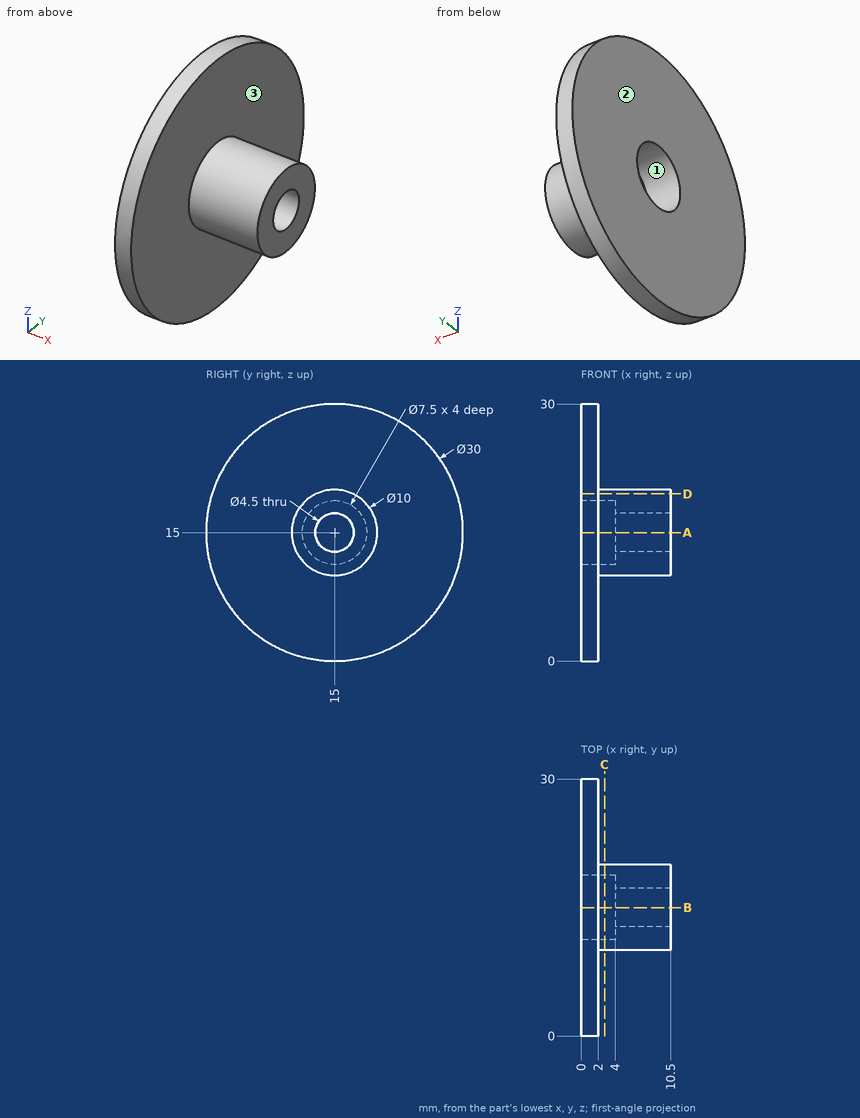
Input: dimensioned drawing with shaded views. Units: mm. Origin: part minimum x, y, z. A direction names the side the tool comes from. Give positions to 0.01 mm unless a question says otherwise; leave off trailing zeros. Order: outer loops, then holes, each group sorted by start corner. A loop starts at its lowest first (then second) coordinate and runs counter-clockwise, first axis right, second up. Notation, with made-up numbers: (-19, 14.5) -> (23, 14.5) arc R22 ccw to (23, 22.5) -> close; hole circle Ø2 at (-24, 2). An arc over 180 degrees is marked (long way). Answer as a JSON object with one key per item and string values.
Q1. First-contact query: pin 1 (1.5 mm diameter, centred on x = 2, y = 5, fed in from +Z); pin 2 (6 mm diameter, centred on x = 4, z = 7, fed in from +Y); pin 3 (5 mm diameter, centred on y = 15, z = 15, fed in from -X); pin 4 (1.5 mm diameter, centred on x = 6, y = 21.5, fed in from +Z). Flat tips, straight axial feed; report the tip coordinate or a pass-through.
Entries:
{"pin 1": "stops at z = 26.81", "pin 2": "stops at y = 28.85", "pin 3": "stops at x = 4", "pin 4": "passes through"}
Q2. Section D-D (z = 19.5). Output: boundary loops of the cut face in (x, y), plus the area to 3 significant figures.
Entries:
{"outline": "(0, 0.69) -> (2, 0.69) -> (2, 12.82) -> (10.5, 12.82) -> (10.5, 17.18) -> (2, 17.18) -> (2, 29.31) -> (0, 29.31) -> close", "area": "94.3 mm^2"}
Q3. Access query for the marked faces 1, 2 and 3. Directions: +Z, -Z, +X, -X, +Y, -Y. A direction counts if a zero-diameter tool reaches every point of the face in a straight line with its end or side. Return the directions, or none.
Entries:
{"face 1": "-X", "face 2": "+Z, -Z, -X, +Y, -Y", "face 3": "+X"}
Q4. Section A-A (z = 15). Output: boundary loops of the cut face in (x, y), plus the area to 4 significant figures.
Entries:
{"outline": "(0, 0) -> (2, 0) -> (2, 10) -> (10.5, 10) -> (10.5, 12.75) -> (4, 12.75) -> (4, 11.25) -> (0, 11.25) -> close; (0, 18.75) -> (4, 18.75) -> (4, 17.25) -> (10.5, 17.25) -> (10.5, 20) -> (2, 20) -> (2, 30) -> (0, 30) -> close", "area": "85.75 mm^2"}
Q5. Material intervals for probe 1 along Z at (x, y) = (2.75, 14.75); probe 2 along Y at (x, z) = (1.95, 15); probe 3 along Y at (x, z) = (8.75, 15), sorted ascending.
Entries:
{"probe 1": "z = 10.01 to 11.26, 18.74 to 19.99", "probe 2": "y = 0 to 11.25, 18.75 to 30", "probe 3": "y = 10 to 12.75, 17.25 to 20"}
Q6. Section C-C (x = 2.75). Output: boundary loops of the cut face in (y, z), plus the area to 3 significant figures.
Entries:
{"outline": "circle Ø10 at (15, 15); hole circle Ø7.5 at (15, 15)", "area": "34.4 mm^2"}
